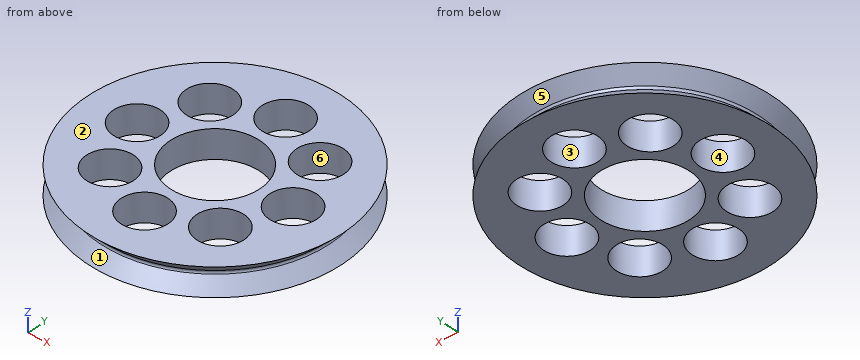
```python
from build123d import *

# Parameters (mm, degrees)
SKETCH_6_R          = 5
CUT_EXTRUDE_2_DEPTH = 10


with BuildPart() as part:
    # 草图2 → 旋转1 (revolve)
    with BuildSketch(Plane(origin=(0, 0, 0), x_dir=(1, 0, 0), z_dir=(0, 1, 0))):
        with BuildLine():
            Line((9.5, 3), (9.5, -3))
            Line((9.5, -3), (27, -3))
            Line((27, -3), (24.353553391, -0.353553391))
            ThreePointArc((24.353553391, -0.353553391), (24.207106781, 0), (24.353553391, 0.353553391))
            Line((24.353553391, 0.353553391), (27, 3))
            Line((27, 3), (9.5, 3))
        make_face()
    revolve(axis=Axis((0, 0, 0), (0, 0, -1)))

    # 草图6 → 切除-拉伸2 (cut)
    with BuildSketch(Plane.XY.offset(3)):
        with Locations((16.5, 0)):
            Circle(SKETCH_6_R)
        with Locations((11.66726189, -11.66726189)):
            Circle(SKETCH_6_R)
        with Locations((0, -16.5)):
            Circle(SKETCH_6_R)
        with Locations((-11.66726189, -11.66726189)):
            Circle(SKETCH_6_R)
        with Locations((-16.5, 0)):
            Circle(SKETCH_6_R)
        with Locations((-11.66726189, 11.66726189)):
            Circle(SKETCH_6_R)
        with Locations((0, 16.5)):
            Circle(SKETCH_6_R)
        with Locations((11.66726189, 11.66726189)):
            Circle(SKETCH_6_R)
    extrude(amount=-CUT_EXTRUDE_2_DEPTH, mode=Mode.SUBTRACT)


solid = part.part
```
Geometry check sheet. Reference: the model listing, model coordinates, mm. Face numbers are marked on the shaded views. A direction names the side the tool comes from. Coordinates: 2 decimals unless noted, no trailing zeros. Order: outer loops, then holes, each group sorted by start corner. A loop starts at its lowest first (then second) coordinate and runs counter-clockwise, first axis right, second up.
Q1. Sectioned sample at C-C on z = 2.3. Give the number of separate pieces and of enclosed holes in the cut face, and give its area (3 significant figures).
Reply:
separate pieces: 1
enclosed holes: 9
area: 1,260 mm2
Q2. Depth check by flat-ended pin: pin 1 Ø3 at (x, y) = (2.5, -7.5) entering from -Z; pin 2 Ø3 at (y, z) = (-19.5, -2.5) entering from +X. Enter the tip coordinate at first touch or a pass-through.
Reply:
pin 1: passes through
pin 2: stops at x = 20.05
Q3. Sectioned sample at A-A on x = 0. Record the cut outline in (y, z), and give its area (3 significant figures).
Reply:
outline: (-27, -3) - (-21.5, -3) - (-21.5, 3) - (-27, 3) - (-24.35, 0.35) arc R0.5 cw to (-24.35, -0.35) - close; (-11.5, -3) - (-9.5, -3) - (-9.5, 3) - (-11.5, 3) - close; (9.5, -3) - (11.5, -3) - (11.5, 3) - (9.5, 3) - close; (21.5, -3) - (27, -3) - (24.35, -0.35) arc R0.5 cw to (24.35, 0.35) - (27, 3) - (21.5, 3) - close
area: 72.1 mm2
Q4. Tool access check on the marked faces 5 and 6. Record the directions out of +Z, -Z, +X, -X, +Y, -Y that give a thin tool (end or side, any length) a straight path to the whole face; none if there is none.
Reply:
face 5: none
face 6: +Z, -Z
Q5. Draft check along Y on the marked faces 1, 2, 3 and 4. Enter one of: released by +Y, released by -Y, zero draft, split by the parting line, or undercut.
Reply:
face 1: split by the parting line
face 2: zero draft
face 3: undercut
face 4: undercut
Q6. Thickness scan on probe 1 along X at (y, z) = (1, -1.2); probe 2 along Y at (x, z) = (14, 1.3); probe 3 along X at (y, z) = (-10, -0.4). Record the ranges inside material, lowest first.
Reply:
probe 1: x = -25.18 to -21.4, -11.6 to -9.45, 9.45 to 11.6, 21.4 to 25.18
probe 2: y = -21.07 to -16.09, -7.24 to -4.33, 4.33 to 7.24, 16.09 to 21.07
probe 3: x = -22.26 to -16.38, -6.95 to 6.95, 16.38 to 22.26
